For this review, take the finished solid that the model builds, in its own axes (mm). A direction names the side the tool comes from. Give positions to 0.01 mm unless a question says otherwise; leave off trailing zeros. Order: outer loops, then holes, each group sorted by start corner. A loop starts at its lowest first (then second) coordinate and runs counter-clockwise, first axis right, second up. Notation, with made-up numbers: (-36, 47.25) - (6, 47.25) arc R10 ccw to (6, 57.25) - close; hole circle Ø10 at (55, -21). An arc over 180 degrees is marked (long way). Put each result on its own line as item: value. Start each with the question number.
```python
from build123d import *

# Parameters (mm, degrees)
SKETCH1_R           = 37
BOSS_EXTRUDE1_DEPTH = 25.05
SKETCH2_R           = 21.5
CUT_EXTRUDE1_DEPTH  = 19.05
SKETCH3_R           = 20.2
CUT_EXTRUDE2_DEPTH  = 4
SKETCH4_R           = 14
CUT_EXTRUDE3_DEPTH  = 58.177814754
SKETCH5_W           = 14
SKETCH5_H           = 14
CUT_EXTRUDE4_DEPTH  = 6
SKETCH6_R           = 1.4
CUT_EXTRUDE5_DEPTH  = 59.01295114
SKETCH7_R           = 1.675
CUT_EXTRUDE6_DEPTH  = 4.75
SKETCH8_R           = 2.2
CUT_EXTRUDE7_DEPTH  = 5.5
SKETCH9_R           = 26
SKETCH9_R_2         = 20.5
CUT_EXTRUDE8_DEPTH  = 1


with BuildPart() as part:
    # Sketch1 → Boss-Extrude1 (new body)
    with BuildSketch(Plane(origin=(0, 0, 0), x_dir=(1, 0, 0), z_dir=(0, 1, 0))):
        with Locations(Location((0, 0, 0), (0, 0, 270))):
            Circle(SKETCH1_R)
    extrude(amount=BOSS_EXTRUDE1_DEPTH)

    # Sketch2 → Cut-Extrude1 (cut)
    with BuildSketch(Plane(origin=(0, 25.05, 0), x_dir=(1, 0, 0), z_dir=(0, 1, 0))):
        with Locations(Location((0, 0, 0), (0, 0, 270))):
            Circle(SKETCH2_R)
    extrude(amount=-CUT_EXTRUDE1_DEPTH, mode=Mode.SUBTRACT)

    # Sketch3 → Cut-Extrude2 (cut)
    with BuildSketch(Plane(origin=(0, 6, 0), x_dir=(1, 0, 0), z_dir=(0, 1, 0))):
        with Locations(Location((0, 0, 0), (0, 0, 270))):
            Circle(SKETCH3_R)
    extrude(amount=-CUT_EXTRUDE2_DEPTH, mode=Mode.SUBTRACT)

    # Sketch4 → Cut-Extrude3 (cut, through all)
    with BuildSketch(Plane(origin=(0, 2, 0), x_dir=(1, 0, 0), z_dir=(0, 1, 0))):
        with Locations(Location((0, 0, 0), (0, 0, 270))):
            Circle(SKETCH4_R)
    extrude(amount=-CUT_EXTRUDE3_DEPTH, mode=Mode.SUBTRACT)

    # Sketch5 → Cut-Extrude4 (cut)
    with BuildSketch(Plane(origin=(0, 0, 0), x_dir=(1, 0, 0), z_dir=(0, 1, 0))):
        with Locations((0, 18)):
            Rectangle(SKETCH5_W, SKETCH5_H)
    extrude(amount=CUT_EXTRUDE4_DEPTH, mode=Mode.SUBTRACT)

    # Sketch6 → Cut-Extrude5 (cut, through all)
    with BuildSketch(Plane(origin=(0, 0, 0), x_dir=(1, 0, 0), z_dir=(0, 1, 0))):
        with Locations(Location((12.021, 12.021, 0), (0, 0, 270))):
            Circle(SKETCH6_R)
        with Locations(Location((12.021, -12.021, 0), (0, 0, 270))):
            Circle(SKETCH6_R)
        with Locations(Location((-12.021, -12.021, 0), (0, 0, 270))):
            Circle(SKETCH6_R)
        with Locations(Location((-12.021, 12.021, 0), (0, 0, 270))):
            Circle(SKETCH6_R)
    extrude(amount=CUT_EXTRUDE5_DEPTH, mode=Mode.SUBTRACT)

    # Sketch7 → Cut-Extrude6 (cut)
    with BuildSketch(Plane(origin=(0, 25.05, 0), x_dir=(1, 0, 0), z_dir=(0, 1, 0))):
        with Locations(Location((27, 0, 0), (0, 0, 270))):
            Circle(SKETCH7_R)
        with Locations(Location((22.713845386, -14.597302071, 0), (0, 0, 270))):
            Circle(SKETCH7_R)
        with Locations(Location((11.216205351, -24.560063875, 0), (0, 0, 270))):
            Circle(SKETCH7_R)
        with Locations(Location((-3.842500633, -26.725178931, 0), (0, 0, 270))):
            Circle(SKETCH7_R)
        with Locations(Location((-17.681239817, -20.405238508, 0), (0, 0, 270))):
            Circle(SKETCH7_R)
        with Locations(Location((-25.906310288, -7.606779035, 0), (0, 0, 270))):
            Circle(SKETCH7_R)
        with Locations(Location((-25.906310288, 7.606779035, 0), (0, 0, 270))):
            Circle(SKETCH7_R)
        with Locations(Location((-17.681239817, 20.405238508, 0), (0, 0, 270))):
            Circle(SKETCH7_R)
        with Locations(Location((-3.842500633, 26.725178931, 0), (0, 0, 270))):
            Circle(SKETCH7_R)
        with Locations(Location((11.216205351, 24.560063875, 0), (0, 0, 270))):
            Circle(SKETCH7_R)
        with Locations(Location((22.713845386, 14.597302071, 0), (0, 0, 270))):
            Circle(SKETCH7_R)
    extrude(amount=-CUT_EXTRUDE6_DEPTH, mode=Mode.SUBTRACT)

    # Sketch8 → Cut-Extrude7 (cut)
    with BuildSketch(Plane(origin=(0, 25.05, 0), x_dir=(1, 0, 0), z_dir=(0, 1, 0))):
        with Locations(Location((31.184102699, 9.154328969, 0), (0, 0, 270))):
            Circle(SKETCH8_R)
        with Locations(Location((-13.503333209, 29.56196868, 0), (0, 0, 270))):
            Circle(SKETCH8_R)
        with Locations(Location((-32.5, 0, 0), (0, 0, 270))):
            Circle(SKETCH8_R)
        with Locations(Location((4.624211408, -32.169343619, 0), (0, 0, 270))):
            Circle(SKETCH8_R)
    extrude(amount=-CUT_EXTRUDE7_DEPTH, mode=Mode.SUBTRACT)

    # Sketch9 → Cut-Extrude8 (cut)
    with BuildSketch(Plane(origin=(0, 0, 0), x_dir=(1, 0, 0), z_dir=(0, 1, 0))):
        with Locations(Location((0, 0, 0), (0, 0, 270))):
            Circle(SKETCH9_R)
        Circle(SKETCH9_R_2, mode=Mode.SUBTRACT)
    extrude(amount=CUT_EXTRUDE8_DEPTH, mode=Mode.SUBTRACT)


solid = part.part
```
1. Clearance check with flat-ended pins moving along their axes: pin 1 (1 mm diameter, centred on x = 0, z = -21.5, fed in from -Y); pin 2 (2 mm diameter, centred on x = 11.22, z = -24.56, fed in from +Y); pin 3 (3 mm diameter, centred on y = 22, z = -27.5, fed in from +X). State where each tip first meets the part, or that it passes through.
2. Add section B-B, the plane x = 0. Give the boundary of the cut face in (y, z).
3. Add section D-D, the plane x = -32.5. Give the boundary of the cut face in (y, z), then the cut area to 3 significant figures.
4. Add section C-C, the plane y = 22.25. Count the separate pieces of the cut face and the enclosed holes in it, then the cut area to 3 significant figures.
5. Tool access review of faces 4 (the face through (-26, 20.3, -8)), 5 (the face through (11.48, 0.99, -10.73)), 6 (the face through (-15.821, 0.493, -20.633)): name each direction out of +Z, -Z, +X, -X, +Y, -Y from which nothing blocks a thin tool from reaching the whole face with its end or side.
6. Wall thickness on line 1 (X direction, y = 21.25, z = 14.5); line 2 (X direction, y = 11.25, z = -1); line 3 (Z direction, x = 15, y = 20.75): over which ranges is each line inside the solid? List them lowest first. Write a range as from..to.
7. The part is to be moulded in two halves that separate along X. For faces 1 (the face through (0, 3, -25)), 2 (the face through (-4, 0, 14)), 3 (the face through (-14.17, 12.35, 34.18)), say which applies: released by +X, released by -X, zero draft, split by the parting line, or undercut.
Found:
1. pin 1: stops at y = 6
1. pin 2: stops at y = 20.3
1. pin 3: stops at x = 26.32
2. outline: (0, -37) - (25.05, -37) - (25.05, -21.5) - (6, -21.5) - (6, -25) - (1, -25) - (1, -26) - (0, -26) - close; (0, 14) - (2, 14) - (2, 20.2) - (6, 20.2) - (6, 21.5) - (25.05, 21.5) - (25.05, 37) - (0, 37) - (0, 26) - (1, 26) - (1, 20.5) - (0, 20.5) - close
3. outline: (0, -17.68) - (25.05, -17.68) - (25.05, -2.2) - (19.55, -2.2) - (19.55, 2.2) - (25.05, 2.2) - (25.05, 17.68) - (0, 17.68) - close
3. area: 862 mm^2
4. separate pieces: 1
4. enclosed holes: 16
4. area: 2,690 mm^2
5. face 4: +Y
5. face 5: +Y, -Y
5. face 6: -Y
6. line 1: x = -34.04..-15.87, 15.87..21.04, 24.39..34.04
6. line 2: x = -36.99..-21.48, 21.48..36.99
6. line 3: z = -33.82..-15.4, 15.4..33.82
7. face 1: undercut
7. face 2: zero draft
7. face 3: split by the parting line
